```python
from build123d import *

# Parameters (mm, degrees)
SKETCH1_R           = 2.5
BOSS_EXTRUDE1_DEPTH = 5
SKETCH2_R           = 1.5
SKETCH2_W           = 50
SKETCH2_H           = 50
CUT_EXTRUDE1_DEPTH  = 5


with BuildPart() as part:
    # Sketch1 → Boss-Extrude1 (new body)
    with BuildSketch(Plane.XY):
        with BuildLine():
            Line((-123.5, 121.5), (-123.5, -121.5))
            ThreePointArc((-123.5, -121.5), (-122.914213562, -122.914213562), (-121.5, -123.5))
            Line((-121.5, -123.5), (121.5, -123.5))
            ThreePointArc((121.5, -123.5), (122.914213562, -122.914213562), (123.5, -121.5))
            Line((123.5, -121.5), (123.5, 121.5))
            ThreePointArc((123.5, 121.5), (122.914213562, 122.914213562), (121.5, 123.5))
            Line((121.5, 123.5), (-121.5, 123.5))
            ThreePointArc((-121.5, 123.5), (-122.914213562, 122.914213562), (-123.5, 121.5))
        make_face()
        with Locations((-118.5, 118.5)):
            Circle(SKETCH1_R, mode=Mode.SUBTRACT)
        with Locations((118.5, 118.5)):
            Circle(SKETCH1_R, mode=Mode.SUBTRACT)
        with Locations((118.5, -118.5)):
            Circle(SKETCH1_R, mode=Mode.SUBTRACT)
        with Locations((-118.5, -118.5)):
            Circle(SKETCH1_R, mode=Mode.SUBTRACT)
    extrude(amount=BOSS_EXTRUDE1_DEPTH)

    # Sketch2 → Cut-Extrude1 (cut)
    with BuildSketch(Plane(origin=(0, 0, 0), x_dir=(-1, 0, 0), z_dir=(0, 0, -1))):
        with Locations((28.284271247, 28.284271247)):
            Circle(SKETCH2_R)
        with Locations((28.284271247, -28.284271247)):
            Circle(SKETCH2_R)
        with Locations((-28.284271247, -28.284271247)):
            Circle(SKETCH2_R)
        with Locations((-28.284271247, 28.284271247)):
            Circle(SKETCH2_R)
        Rectangle(SKETCH2_W, SKETCH2_H)
    extrude(amount=-CUT_EXTRUDE1_DEPTH, mode=Mode.SUBTRACT)


solid = part.part
```
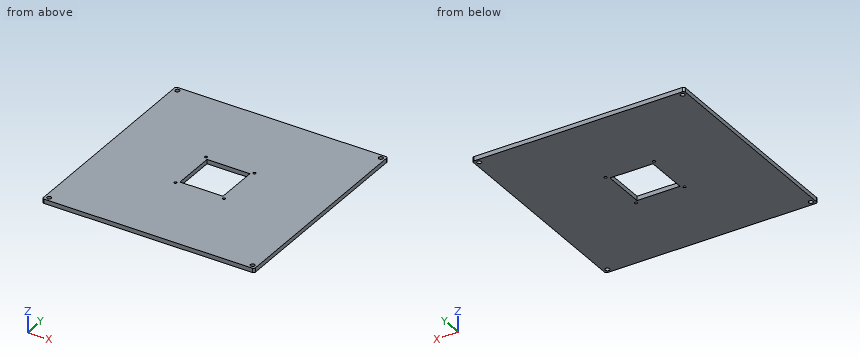
CAD build for the part. Positions are in the model's coordinates, mm. Coordinates: 2 decimals unless noted, no trailing zeros. Write each loop counter-clockwise with the first axis right and the second up, starting at its lowest first coordinate (ties: lowest second). Pieces come first, ordered by that corner, then holes. Notation, with made-up numbers: (8, 46.25) -> (32, 46.25) arc R26 ccw to (32, 61.25) -> close; hole circle Ø7 at (83, -38.5). An arc over 180 degrees is marked (long way). Return JSON: item names as keys, results as strings. Group by question number.
Q1. Cut at A-A, the plane x = -10.5. Give the cut face in (y, z), then the cut area to 3 significant figures.
Q2. Flat gauge pin, fed straight in: pin 1 (6.5 mm diameter, centred on x = 118.5, y = 118.5, fed in from -Z). Where does the tip first touch, or does it go through?
Q3. Drill centre lines: line 1 (Y direction, x = -118.5, z = 3.05); line 2 (Y direction, x = -12, z = 3.9). Where is each one in solid material? Low to high.
Returned:
{
 "1": {"outline": "(-123.5, 0) -> (-25, 0) -> (-25, 5) -> (-123.5, 5) -> close; (25, 0) -> (123.5, 0) -> (123.5, 5) -> (25, 5) -> close", "area": "985 mm2"},
 "2": {"pin 1": "stops at z = 0"},
 "3": {"line 1": "y = -123.5 to -121, -116 to 116, 121 to 123.5", "line 2": "y = -123.5 to -25, 25 to 123.5"}
}
